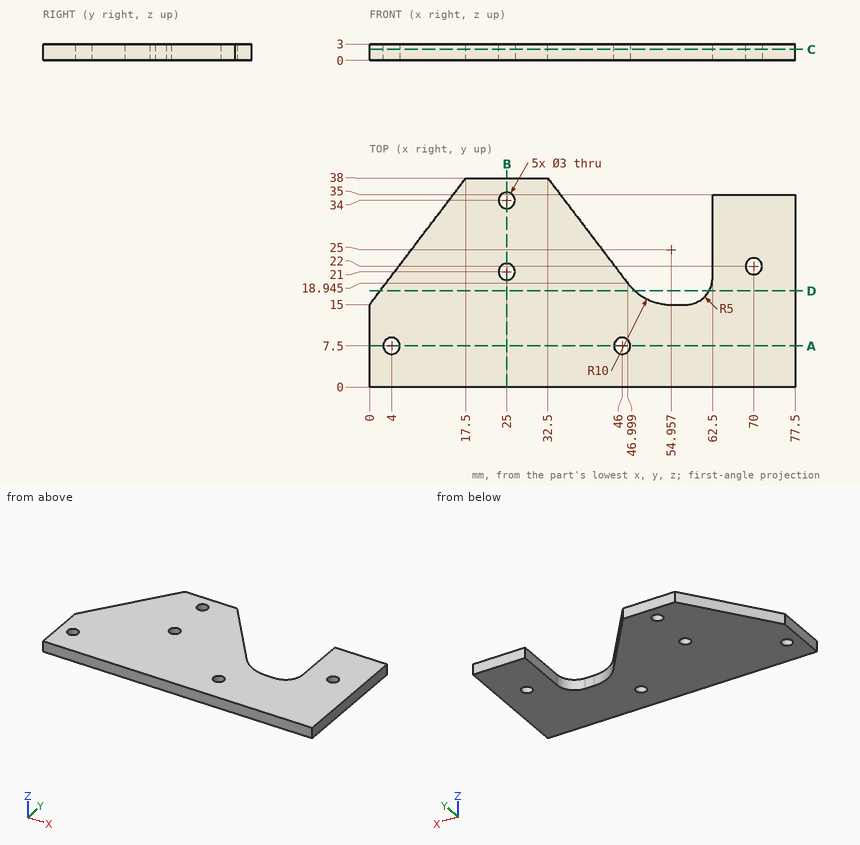
Geometry: see drawing. Coordinates: mm, zero at the bounding-box minimum. Round coordinates to 2 decimals unless told otherwise and drop trailing zeros. Write each loop counter-clockwise with the first axis right and the second up, starting at its lowest first coordinate (ties: lowest second). Pieces come first, ordered by that corner, then holes. Notation, with made-up numbers: (47, 21) -> (51, 21) arc R25 ccw to (51, 41) -> close; hole circle Ø6 at (-25.75, -2). An arc over 180 degrees is marked (long way). Answer as CSV lines item,"result".
1. Ray query, L1, parallel to Y at x = 25, z = 2.2; L2, parallel to Y at x = 70, z = 1; L3, parallel to Y at x = 45, z = 2 (1 decimal). Return the intervals inside material, ascending. Write a range as [from, to].
Geometry says:
L1,"y = [0, 19.5], [22.5, 32.5], [35.5, 38]"
L2,"y = [0, 20.5], [23.5, 35]"
L3,"y = [0, 6.4], [8.6, 21.6]"
2. Section D-D (y = 17.5). Return the cut outline in (x, z), plus the area to 3 significant figures.
Geometry says:
outline,"(1.9, 0) -> (48.34, 0) -> (48.34, 3) -> (1.9, 3) -> close; (61.83, 0) -> (77.5, 0) -> (77.5, 3) -> (61.83, 3) -> close"
area,"186 mm^2"
3. Contact query for flat-ended pins moving along their axis: P1, Ø1.5, axis at x = 68.5, z = 2, coming from the +Y side; P2, Ø0.8, axis at x = 57, z = 2, coming from the +Y side; P3, Ø12, axis at x = 42.5, y = 27, coming from the -Z side. Output: stop coordinate, or through.
Geometry says:
P1,"stops at y = 35"
P2,"stops at y = 15"
P3,"stops at z = 0"
4. Section A-A (y = 7.5). Return the cut outline in (x, z).
Geometry says:
outline,"(0, 0) -> (2.5, 0) -> (2.5, 3) -> (0, 3) -> close; (5.5, 0) -> (44.5, 0) -> (44.5, 3) -> (5.5, 3) -> close; (47.5, 0) -> (77.5, 0) -> (77.5, 3) -> (47.5, 3) -> close"
5. Section C-C (z = 2). Return the cut outline in (x, y) (1 decimal), plus the area to 3 significant figures.
Geometry says:
outline,"(0, 0) -> (77.5, 0) -> (77.5, 35) -> (62.5, 35) -> (62.5, 20) arc R5 cw to (57.5, 15) -> (55, 15) arc R10 cw to (47, 18.9) -> (32.5, 38) -> (17.5, 38) -> (0, 15) -> close; hole circle Ø3 at (4, 7.5); hole circle Ø3 at (25, 21); hole circle Ø3 at (25, 34); hole circle Ø3 at (46, 7.5); hole circle Ø3 at (70, 22)"
area,"2,180 mm^2"
6. Section B-B (x = 25). Return the cut outline in (y, z).
Geometry says:
outline,"(0, 0) -> (19.5, 0) -> (19.5, 3) -> (0, 3) -> close; (22.5, 0) -> (32.5, 0) -> (32.5, 3) -> (22.5, 3) -> close; (35.5, 0) -> (38, 0) -> (38, 3) -> (35.5, 3) -> close"
